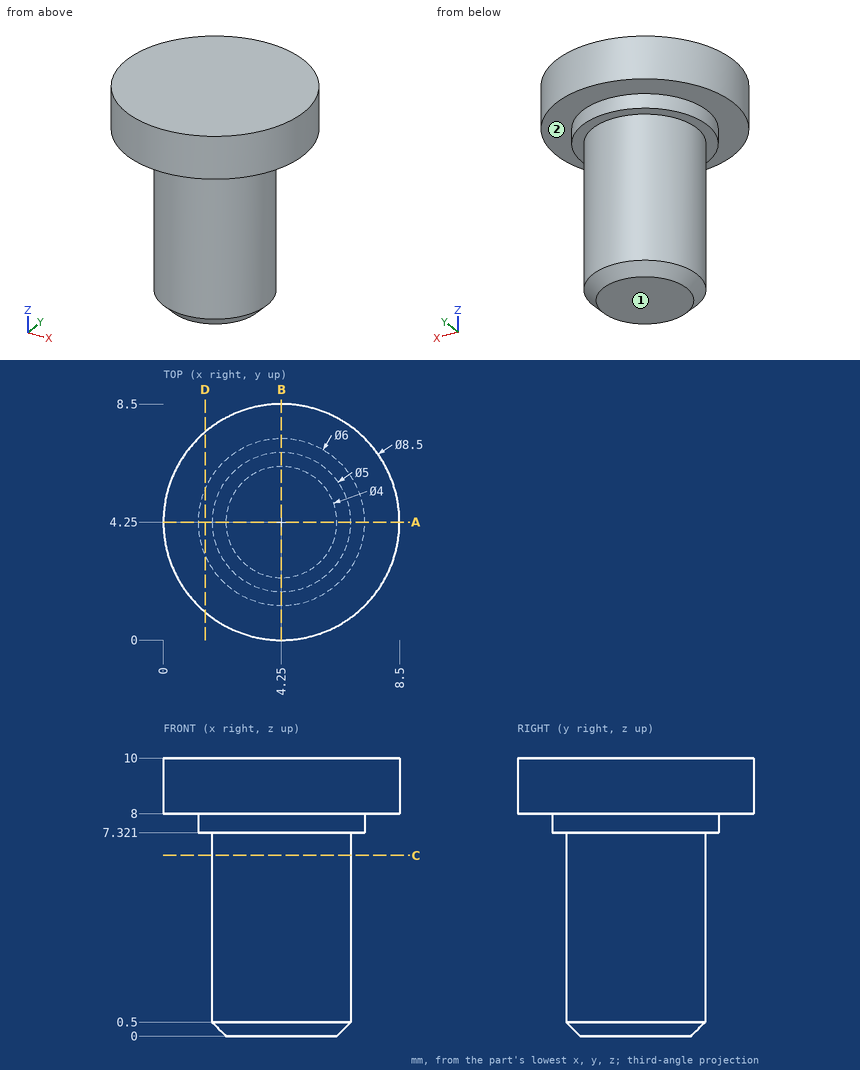
The drawing under review shows one solid part. Ordinate dimensions are in mm from its lowest x, y, z. A direction names the side the tool comes from. Coordinates: 2 decimals unless noted, no trailing zeros. Write each loop counter-clockwise with the first axis right and the second up, starting at its lowest first coordinate (ties: lowest second). Pieces come first, ordered by that corner, then holes. Notation, with made-up numbers: (48, -17.5) - (98, -17.5) arc R12 ccw to (98, -8.5) - close; hole circle Ø4 at (58, 81.5). An arc over 180 degrees is marked (long way). Put each result on its own line as item: value.
1. Add section C-C, the plane z = 6.5. Give the boundary of the cut face in (x, y), then the cut area to 3 significant figures.
Values found:
outline: circle Ø5 at (4.25, 4.25)
area: 19.6 mm²
2. Machinability: for the marked faces 1 and 2, which of the approach directions +Z, -Z, +X, -X, +Y, -Y give a long, thin tool a straight path to every point of the face, cutting with its end or side? Answer none if there is none.
Values found:
face 1: -Z, +X, -X, +Y, -Y
face 2: -Z
3. Add section A-A, the plane y = 4.25. Give the boundary of the cut face in (x, z), then the cut area to 3 significant figures.
Values found:
outline: (0, 8) - (1.25, 8) - (1.25, 7.32) - (1.75, 7.32) - (1.75, 0.5) - (2.25, 0) - (6.25, 0) - (6.75, 0.5) - (6.75, 7.32) - (7.25, 7.32) - (7.25, 8) - (8.5, 8) - (8.5, 10) - (0, 10) - close
area: 57.4 mm²
4. Add section D-D, the plane x = 1.5. Give the boundary of the cut face in (y, z).
Values found:
outline: (1.01, 8) - (3.05, 8) - (3.05, 7.32) - (5.45, 7.32) - (5.45, 8) - (7.49, 8) - (7.49, 10) - (1.01, 10) - close
5. For pin 1 (3 mm diameter, centred on x = 5, y = 3.5, fed in from -Z); pin 2 (1 mm diameter, centred on x = 5.5, z = 2, fed in from -Y) (1 decimal); pin 3 (1.5 mm diameter, centred on x = 6.5, z = 6, fed in from +Y), all flat-tipped, find the tip position at first contact; note any pin that passes through.
Values found:
pin 1: z = 0
pin 2: y = 1.9
pin 3: y = 6.25
6. Wall thickness on probe 1 along Z at (x, y) = (1.75, 1.25); probe 2 along X at (y, z) = (5.75, 2.5); probe 3 along Y at (x, z) = (4.25, 3.75): over which ranges is each line inside the solid? List them lowest first.
Values found:
probe 1: 8 to 10
probe 2: 2.25 to 6.25
probe 3: 1.75 to 6.75
